Geometry check sheet. Reference: the model listing, model coordinates, mm. A direction names the side the tool comes from. Give positions to 0.01 mm unless a question says otherwise; leave off trailing zeros. Write each loop counter-clockwise with the first axis right and the second up, starting at its lowest first coordinate (ties: lowest second). Pieces come first, ordered by that corner, then holes.
(1) Thickness scan on line 1 along Z through (x, y) = (-54, 132); line 2 along X through (y, z) = (44, 18); line 3 along X through (y, z) = (26.5, -319). Record the ranges inside material, lowest first.
(2) Tool access check on faces 1 (the flat face through (-319, 40, -368)), 2 (the flat face through (-160, -216, -200)), 3 (the flat face through (78.7, 171.9, -17.3)), 4 (the flat face through (-330.24, 20.28, 386.63)), 5 (the flat face through (-309, 0, -369)). Record the directions out of +Z, -Z, +X, -X, +Y, -Y that give a thin tool (end or side, any length) a straight path to the whole face; none if there is none.
(3) Cross-section at B-B (z = -113). Count the separate pieces of the cut face and the enclosed holes in it, and give its area (3 significant figures).
(4) Cross-section at A-A (y = 110.5). Record the boundary of the cut face in (x, z).
(5) Mould release check, pull along Y, two halves, no side actions. Record for faces 6 (the flat face through (-327, -20, -376)), 7 (the flat face through (-320, 40, 369)), 8 (the flat face through (302.54, 19.72, -379.21)): +Y half, -Y half, draft (parallel to the pull), parting line (faces both ways), or undercut.
(6) Depth check by flat-ended pin: P1, Ø2, axis at y = -46, z = -99, coming from the +X side; P2, Ø3, axis at x = -5, y = -127.5, coming from the +Z side; P3, Ø16.5, axis at x = -331.5, z = -370, coming from the -Y side. Enter the tip coordinate at first touch or a pass-through.
```python
from build123d import *

# Parameters (mm, degrees)
SKETCH_9_W            = 300
SKETCH_9_H            = 150
EXTRUDE_2_DEPTH       = 162
EXTRUDE_3_DEPTH       = 340
EXTRUDE_3_DEPTH_BACK  = 20
SKETCH_10_R           = 12
EXTRUDE_4_DEPTH       = 338.918510241
EXTRUDE_4_DEPTH_BACK  = 20
SKETCH_11_R           = 12
EXTRUDE_5_DEPTH       = 340
EXTRUDE_5_DEPTH_BACK  = 20
SKETCH_13_R           = 12
EXTRUDE_6_DEPTH       = 340
EXTRUDE_6_DEPTH_BACK  = 20
SKETCH_12_R           = 12
EXTRUDE_7_DEPTH       = 20
EXTRUDE_7_DEPTH_BACK  = 20
SKETCH_14_W           = 40
SKETCH_14_H           = 40
EXTRUDE_8_DEPTH       = 20
EXTRUDE_8_DEPTH_BACK  = 20
SKETCH_17_W           = 40
SKETCH_17_H           = 40
EXTRUDE_9_DEPTH       = 20
EXTRUDE_9_DEPTH_BACK  = 20
SKETCH_18_W           = 40
SKETCH_18_H           = 40
EXTRUDE_10_DEPTH      = 20
EXTRUDE_10_DEPTH_BACK = 20
SKETCH_20_W           = 40
SKETCH_20_H           = 40
EXTRUDE_11_DEPTH      = 20
EXTRUDE_11_DEPTH_BACK = 20
SKETCH_21_R           = 10
SKETCH_22_R           = 35
EXTRUDE_12_DEPTH      = 20
EXTRUDE_13_DEPTH      = 250
EXTRUDE_13_DEPTH_BACK = 20
SKETCH_23_R           = 12
EXTRUDE_14_DEPTH      = 250
EXTRUDE_14_DEPTH_BACK = 20
SKETCH_24_R           = 12
EXTRUDE_15_DEPTH      = 20
EXTRUDE_15_DEPTH_BACK = 20
EXTRUDE_16_DEPTH      = 160
EXTRUDE_16_DEPTH_BACK = 160
SKETCH_29_R           = 12


with BuildPart() as part:
    # 草图9 → 凸台-拉伸2 (new body)
    with BuildSketch(Plane(origin=(0, 0, 0), x_dir=(1, 0, 0), z_dir=(0, 1, 0))):
        Rectangle(SKETCH_9_W, SKETCH_9_H)
    extrude(amount=EXTRUDE_2_DEPTH)

    # 草图10 → 凸台-拉伸3 (add, two sides: drawn at the far end of the back side and taken through both)
    with BuildSketch(Plane(origin=(-69.975952642, 0, 121.201905284), x_dir=(0, -1, 0), z_dir=(-0.500000000000001, 0, 0.866025403784438)).offset(-EXTRUDE_3_DEPTH_BACK)):
        with Locations(Location((-20, -92.403810568, 0), (0, 0, 90))):
            Circle(SKETCH_10_R)
    extrude(amount=EXTRUDE_3_DEPTH + EXTRUDE_3_DEPTH_BACK)

    # 草图11 → 凸台-拉伸4 (add, two sides: drawn at the far end of the back side and taken through both)
    with BuildSketch(Plane(origin=(-69.975952642, 0, -121.201905284), x_dir=(0, -1, 0), z_dir=(-0.5000000000000011, 0, -0.866025403784438)).offset(-EXTRUDE_4_DEPTH_BACK)):
        with Locations(Location((-20, 92.403810568, 0), (0, 0, 90))):
            Circle(SKETCH_11_R)
    extrude(amount=EXTRUDE_4_DEPTH + EXTRUDE_4_DEPTH_BACK)

    # 草图13 → 凸台-拉伸5 (add, two sides: drawn at the far end of the back side and taken through both)
    with BuildSketch(Plane(origin=(69.975952642, 0, 121.201905284), x_dir=(0, -1, 0), z_dir=(0.5000000000000011, 0, 0.866025403784438)).offset(-EXTRUDE_5_DEPTH_BACK)):
        with Locations(Location((-20, 92.403810568, 0), (0, 0, 90))):
            Circle(SKETCH_13_R)
    extrude(amount=EXTRUDE_5_DEPTH + EXTRUDE_5_DEPTH_BACK)

    # 草图12 → 凸台-拉伸6 (add, two sides: drawn at the far end of the back side and taken through both)
    with BuildSketch(Plane(origin=(69.975952642, 0, -121.201905284), x_dir=(0, -1, 0), z_dir=(0.5000000000000009, 0, -0.866025403784438)).offset(-EXTRUDE_6_DEPTH_BACK)):
        with Locations(Location((-20, -92.403810568, 0), (0, 0, 90))):
            Circle(SKETCH_12_R)
    extrude(amount=EXTRUDE_6_DEPTH + EXTRUDE_6_DEPTH_BACK)

    # 草图14 → 凸台-拉伸7 (add, two sides: drawn at the far end of the back side and taken through both)
    with BuildSketch(Plane(origin=(-239.975952642, 0, 415.650542571), x_dir=(0.8660254037844382, 0, 0.500000000000001), z_dir=(-0.500000000000001, 0, 0.8660254037844382)).offset(-EXTRUDE_7_DEPTH_BACK)):
        with Locations((-92.403810568, 20)):
            Rectangle(SKETCH_14_W, SKETCH_14_H)
    extrude(amount=EXTRUDE_7_DEPTH + EXTRUDE_7_DEPTH_BACK)

    # 草图17 → 凸台-拉伸8 (add, two sides: drawn at the far end of the back side and taken through both)
    with BuildSketch(Plane(origin=(-239.435207762, 0, -414.713944965), x_dir=(-0.866025403784438, 0, 0.5000000000000012), z_dir=(-0.5000000000000011, 0, -0.8660254037844379)).offset(-EXTRUDE_8_DEPTH_BACK)):
        with Locations((92.403810568, 20)):
            Rectangle(SKETCH_17_W, SKETCH_17_H)
    extrude(amount=EXTRUDE_8_DEPTH + EXTRUDE_8_DEPTH_BACK)

    # 草图18 → 凸台-拉伸9 (add, two sides: drawn at the far end of the back side and taken through both)
    with BuildSketch(Plane(origin=(239.975952642, 0, -415.650542571), x_dir=(-0.866025403784438, 0, -0.5000000000000012), z_dir=(0.5000000000000011, 0, -0.8660254037844379)).offset(-EXTRUDE_9_DEPTH_BACK)):
        with Locations((-92.403810568, 20)):
            Rectangle(SKETCH_18_W, SKETCH_18_H)
    extrude(amount=EXTRUDE_9_DEPTH + EXTRUDE_9_DEPTH_BACK)

    # 草图20 → 凸台-拉伸10 (add, two sides: drawn at the far end of the back side and taken through both)
    with BuildSketch(Plane(origin=(239.975952642, 0, 415.650542571), x_dir=(0.866025403784438, 0, -0.5000000000000012), z_dir=(0.5000000000000011, 0, 0.8660254037844379)).offset(-EXTRUDE_10_DEPTH_BACK)):
        with Locations((92.403810568, 20)):
            Rectangle(SKETCH_20_W, SKETCH_20_H)
    extrude(amount=EXTRUDE_10_DEPTH + EXTRUDE_10_DEPTH_BACK)

    # 草图21 → 凸台-拉伸11 (add, two sides: drawn at the far end of the back side and taken through both)
    with BuildSketch(Plane.XZ.offset(-EXTRUDE_11_DEPTH_BACK)):
        with Locations(Location((-320, 369.448637287, 0), (0, 0, 270))):
            Circle(SKETCH_21_R)
        with Locations(Location((-319.45925512, -368.512039681, 0), (0, 0, 270))):
            Circle(SKETCH_21_R)
        with Locations(Location((320, -369.448637287, 0), (0, 0, 270))):
            Circle(SKETCH_21_R)
        with Locations(Location((320, 369.448637287, 0), (0, 0, 270))):
            Circle(SKETCH_21_R)
    extrude(amount=EXTRUDE_11_DEPTH + EXTRUDE_11_DEPTH_BACK)

    # 草图22 → 凸台-拉伸12 (add)
    with BuildSketch(Plane.XZ.offset(20)):
        with Locations(Location((-319.45925512, -368.512039681, 0), (0, 0, 270))):
            Circle(SKETCH_22_R)
        with Locations(Location((320, -369.448637287, 0), (0, 0, 270))):
            Circle(SKETCH_22_R)
        with Locations(Location((320, 369.448637287, 0), (0, 0, 270))):
            Circle(SKETCH_22_R)
        with Locations(Location((-319.45925512, 369.448637287, 0), (0, 0, 270))):
            Circle(SKETCH_22_R)
    extrude(amount=EXTRUDE_12_DEPTH)

    # 草图23 → 凸台-拉伸13 (add, two sides: drawn at the far end of the back side and taken through both)
    with BuildSketch(Plane(origin=(0, -32.475952642, 18.75), x_dir=(1, 0, 0), z_dir=(0, -0.866025403784438, 0.500000000000001)).offset(-EXTRUDE_13_DEPTH_BACK)):
        with Locations(Location((0, 64.951905284, 0), (0, 0, 270))):
            Circle(SKETCH_23_R)
    extrude(amount=EXTRUDE_13_DEPTH + EXTRUDE_13_DEPTH_BACK)

    # 草图24 → 凸台-拉伸14 (add, two sides: drawn at the far end of the back side and taken through both)
    with BuildSketch(Plane(origin=(0, -32.475952642, -18.75), x_dir=(-1, 0, 0), z_dir=(0, -0.866025403784438, -0.500000000000001)).offset(-EXTRUDE_14_DEPTH_BACK)):
        with Locations(Location((0, 64.951905284, 0), (0, 0, 90))):
            Circle(SKETCH_24_R)
    extrude(amount=EXTRUDE_14_DEPTH + EXTRUDE_14_DEPTH_BACK)

    # 草图26 → 凸台-拉伸15 (add, two sides: drawn at the far end of the back side and taken through both)
    with BuildSketch(Plane(origin=(0, 162, 0), x_dir=(1, 0, 0), z_dir=(0, 1, 0)).offset(-EXTRUDE_15_DEPTH_BACK)):
        Polygon((100, 5.002088535), (56.698729811, 30.002088535), (56.698729811, -19.997911465), align=None)
    extrude(amount=EXTRUDE_15_DEPTH + EXTRUDE_15_DEPTH_BACK)

    # 草图29 → 凸台-拉伸16 (add, two sides: drawn at the far end of the back side and taken through both)
    with BuildSketch(Plane.ZY.offset(-EXTRUDE_16_DEPTH_BACK)):
        with Locations((-200, -216.506350946)):
            Circle(SKETCH_29_R)
        with Locations((200, -216.506350946)):
            Circle(SKETCH_29_R)
    extrude(amount=EXTRUDE_16_DEPTH + EXTRUDE_16_DEPTH_BACK)


solid = part.part
```
Reply:
1. line 1: z = -75 to 75
1. line 2: x = -150 to 150
1. line 3: x = -302.52 to -279.23, 279.23 to 302.52
2. face 1: +Z, -Z, +X, -X, +Y
2. face 2: +Z, -Z, -X, +Y, -Y
2. face 3: -Z, +X, +Y
2. face 4: +Z, -X, +Y
2. face 5: none
3. separate pieces: 3
3. enclosed holes: 0
3. area: 1,950 mm2
4. outline: (-150, -75) - (150, -75) - (150, 75) - (-150, 75) - close
5. face 6: undercut
5. face 7: +Y half
5. face 8: draft
6. P1: stops at x = 11.94
6. P2: stops at z = 162.33
6. P3: stops at y = -40
